Geometry check sheet. Reference: the model listing, model coordinates, mm. A direction names the side the tool comes from. Round coordinates to 2 decimals unless told otherwise and drop trailing zeros. Order: outer loops, then holes, each group sorted by start corner. A loop starts at its lowest first (then second) coordinate and runs counter-clockwise, first axis right, second up.
(1) Sectioned sample at A-A (x = 24). Record the boundary of the cut face in (y, z), plus the area to 3 significant figures.
(2) Go/stop test with flat-tipped pins: pin 1 (6 mm diameter, centred on x = 10.5, y = 18, fed in from -Z); pin 2 (23.5 mm diameter, centred on y = 0, z = 0, fed in from -X); pin 3 (8 mm diameter, centred on x = -13, y = 15, fed in from -Z); pin 4 (2 mm diameter, centred on x = -9.5, y = 5, fed in from +Z). Record where each tip stops, or that it passes through.
(3) Sectioned sample at C-C (y = -17). Record the boundary of the cut face in (x, z), plus the area to 3 significant figures.
(4) Set-up check for faces 1 (the face through (-15, -15, 5)), 2 (the face through (18.899, -7.91, -10.316)), 3 (the face through (15, -15, -5)): record each of +Z, -Z, +X, -X, +Y, -Y from which the full face is reachable in a straight line by a thin tool's end or side.
(5) Sectioned sample at B-B (x = 12). Record the boundary of the cut face in (y, z).
(6) Release check for a two-part mould opening along Y. For faces 4 (the face through (-18.584, -7.91, -10.316)), 5 (the face through (-0.21, 22.804, -2.994)), 6 (the face through (-30, 13.4, -0.1)) record: +Y half, -Y half, draft (parallel to the pull), parting line (faces both ways), or undercut.
(7) Material ranges on line 1 along Y through (x, z) = (-17.75, 0); line 2 along X through (y, z) = (-12.5, 9.5); line 3 along Z through (x, y) = (0.5, -6), recorded low to high.
from build123d import *


with BuildPart() as f1:
    # F0 (on Front) → F1 (revolve)
    with BuildSketch(Plane.XZ):
        with BuildLine():
            Line((-30, 13), (-7.483315, 13))
            ThreePointArc((-7.483315, 13), (0, 15), (7.483315, 13))
            Line((7.483315, 13), (30, 13))
            Line((30, 13), (30, 15))
            Line((30, 15), (15, 15))
            Line((15, 15), (15, 23))
            Line((15, 23), (-15, 23))
            Line((-15, 23), (-15, 15))
            Line((-15, 15), (-30, 15))
            Line((-30, 15), (-30, 13))
        make_face()
    revolve(axis=Axis((-26.536044, 0, 0), (-1, 0, 0)))


solid = f1.part
Answer below:
1. outline: circle Ø30 at (0, 0); hole circle Ø26 at (0, 0)
1. area: 176 mm2
2. pin 1: stops at z = -17.44
2. pin 2: passes through
2. pin 3: stops at z = -20.2
2. pin 4: stops at z = 22.65
3. outline: (-15, -15.49) - (15, -15.49) - (15, 15.49) - (-15, 15.49) - close
3. area: 930 mm2
4. face 1: -X
4. face 2: +X, -X
4. face 3: +X
5. outline: circle Ø46 at (0, 0); hole circle Ø26 at (0, 0)
6. face 4: undercut
6. face 5: parting line
6. face 6: draft
7. line 1: y = -15 to -13, 13 to 15
7. line 2: x = -15 to 15
7. line 3: z = -22.2 to -13.74, 13.74 to 22.2
